```python
from build123d import *

# Parameters (mm, degrees)
SKETCH1_R           = 1.6
BOSS_EXTRUDE1_DEPTH = 3
CHAMFER1_SIZE       = 1.6
FILLET1_R           = 10
SKETCH2_W           = 17.95
SKETCH2_H           = 5.409714066
CUT_EXTRUDE1_DEPTH  = 1


with BuildPart() as part:
    # Sketch1 → Boss-Extrude1 (new body)
    with BuildSketch(Plane(origin=(0, 0, 0), x_dir=(1, 0, 0), z_dir=(0, 1, 0))):
        with BuildLine():
            Line((8.827855615, 2), (-8.827855615, 2))
            ThreePointArc((-8.827855615, 2), (-15.75, 0), (-8.827855615, -2))
            Line((-8.827855615, -2), (8.827855615, -2))
            ThreePointArc((8.827855615, -2), (15.75, 0), (8.827855615, 2))
        make_face()
        with Locations(Location((-12, 0, 0), (0, 0, 270))):
            Circle(SKETCH1_R, mode=Mode.SUBTRACT)
        with Locations(Location((12, 0, 0), (0, 0, 270))):
            Circle(SKETCH1_R, mode=Mode.SUBTRACT)
    extrude(amount=BOSS_EXTRUDE1_DEPTH)

    # Chamfer1
    chamfer1_edges = [part.edges().sort_by_distance(p)[0] for p in [
        (12, 3, -1.6),
        (-12, 3, -1.6),
    ]]
    chamfer(chamfer1_edges, length=CHAMFER1_SIZE)

    # Fillet1
    fillet1_edges = [part.edges().sort_by_distance(p)[0] for p in [
        (-8.827855615, 1.5, -2),
        (8.827855615, 1.5, -2),
        (8.827855615, 1.5, 2),
        (-8.827855615, 1.5, 2),
    ]]
    fillet(fillet1_edges, radius=FILLET1_R)

    # Sketch2 → Cut-Extrude1 (cut)
    with BuildSketch(Plane(origin=(0, 0, 0), x_dir=(-1, 0, 0), z_dir=(0, -1, 0))):
        Rectangle(SKETCH2_W, SKETCH2_H)
    extrude(amount=-CUT_EXTRUDE1_DEPTH, mode=Mode.SUBTRACT)


solid = part.part
```
Work out the finished part from the listing and answer in its coordinate system (mm). A direction names the side the tool comes from. Give positions to 0.01 mm unless a question says otherwise; leave off trailing zeros. Write each loop counter-clockwise with the first axis right and the second up, starting at its lowest first coordinate (ties: lowest second). Pieces come first, ordered by that corner, then holes.
(1) The part is cut by section A-A on x = -12. Write down the section's boundary in (y, z), plus the area to 3 significant figures.
Final values:
outline: (0, -3.75) - (3, -3.75) - (3, -3.2) - (1.4, -1.6) - (0, -1.6) - close; (0, 1.6) - (1.4, 1.6) - (3, 3.2) - (3, 3.75) - (0, 3.75) - close
area: 10.3 mm2
(2) The part is cut by section C-C on y = 0.6. Write down the section's boundary in (x, z) (3 decimals), plus the area to 3 significant figures.
Final values:
outline: (-10.169, -3.273) arc R10 cw to (-8.975, -2.705) - (-8.975, 2.705) arc R10 cw to (-10.169, 3.273) arc R3.75 ccw (long way) to start; (8.975, -2.705) arc R10 cw to (10.169, -3.273) arc R3.75 ccw (long way) to (10.169, 3.273) arc R10 cw to (8.975, 2.705) - close; hole circle Ø3.2 at (-12, 0); hole circle Ø3.2 at (12, 0)
area: 68.6 mm2
(3) The part is cut by section B-B on z = 0. Write down the section's boundary in (x, y) (3 decimals).
Final values:
outline: (-15.75, 0) - (-13.6, 0) - (-13.6, 1.4) - (-15.2, 3) - (-15.75, 3) - close; (-10.4, 0) - (-8.975, 0) - (-8.975, 1) - (8.975, 1) - (8.975, 0) - (10.4, 0) - (10.4, 1.4) - (8.8, 3) - (-8.8, 3) - (-10.4, 1.4) - close; (13.6, 0) - (15.75, 0) - (15.75, 3) - (15.2, 3) - (13.6, 1.4) - close
(4) Flat-ended cylindrical pins translate along their axes: pin 1 Ø2.5 at (x, z) = (-2, 1) entering from -Y; pin 2 Ø1.6 at (x, y) = (-0.5, 2) entering from +Z; pin 3 Ø0.8 at (y, z) = (0.5, 1) entering from +X. Find the tip coordinate at first contact, or state that the pin passes through.
Final values:
pin 1: stops at y = 1
pin 2: stops at z = 2
pin 3: stops at x = 15.7
(5) The mould has two halves that part along Z. Classify faces 6 (the cylindrical face through (-13.56, 0.69, -0.35)), 7 (the cylindrical face through (-7.775, 1.854, -2.314)), 8 (the cylindrical face through (13.586, 0.69, -0.208)), 9 (the flat face through (8.975, 0.5, 0)): pulls with the +Z half, pulls with the -Z half, needs draft (parallel to the pull), parting line crosses it, or undercut.
Final values:
face 6: undercut
face 7: pulls with the -Z half
face 8: undercut
face 9: needs draft
(6) Straight lines are drawn through the part: line 1 (X direction, y = 0.8, z = 0) (3 decimals); line 2 (X direction, y = 1.1, z = 0); line 3 (X direction, y = 1.85, z = 0.5). For each, find the intervals that lie inside material, in ascending order.
Final values:
line 1: x = -15.75 to -13.6, -10.4 to -8.975, 8.975 to 10.4, 13.6 to 15.75
line 2: x = -15.75 to -13.6, -10.4 to 10.4, 13.6 to 15.75
line 3: x = -15.72 to -13.99, -10.01 to 10.01, 13.99 to 15.72
(7) The part is cut by section D-D on y = 1.9. Write down the section's boundary in (x, z).
Final values:
outline: (-10.17, -3.27) arc R10 cw to (-5.29, -2) - (5.29, -2) arc R10 cw to (10.17, -3.27) arc R3.75 ccw (long way) to (10.17, 3.27) arc R10 cw to (5.29, 2) - (-5.29, 2) arc R10 cw to (-10.17, 3.27) arc R3.75 ccw (long way) to start; hole circle Ø4.2 at (-12, 0); hole circle Ø4.2 at (12, 0)
(8) Which of the six approach directions +Z, -Z, +X, -X, +Y, -Y give full straight-line access (tool end or side, diameter ignored) to faces 1 (the cylindrical face through (7.84, 1.85, 2.33)), 2 (the cylindrical face through (15.75, 1.48, 0.11)), 3 (the flat face through (0, 3, 0)), 4 (the flat face through (0, 1, 0)), 5 (the cylindrical face through (7.775, 1.854, -2.314))?
Final values:
face 1: +Z, +Y, -Y
face 2: +Y, -Y
face 3: +Z, -Z, +X, -X, +Y
face 4: +Z, -Z, -Y
face 5: -Z, +Y, -Y
